Can you work these out from the drawing? Everything is in mm from the part's minimum corner. Give positions to 0.01 mm unless a question says otherwise; leave off trailing zeros. Order: outer loops, then holes, each group sorted by start corner. A loop starts at its lowest first (then second) coordinate and runs counter-clockwise, first axis right, second up. Notation, with made-up numbers: (88.25, 0) -> (133.25, 0) arc R21 ccw to (133.25, 10) -> close; hole circle Ø10 at (-29.5, 83.25). An arc over 180 degrees is marked (long way). Answer as CSV lines item,"result". Start each with the question number.
(1) I want a section at A-A (x = 8.5). Please give me the cut outline in (y, z) (1 decimal).
(2) Will this pin go through, and if not, where does the flat tip stop? pin 1 Ø3.5 at (x, z) = (4.5, 43.5) entering from -Y.
(3) I need wall thicknesses on L1, parallel to Z at x = 9.5, y = 1 (1 decimal); L2, parallel to Z at x = 13.5, y = 0.5 (1 decimal); L3, parallel to X at y = 0.5, z = 50 (1 decimal). Which ranges of each line are inside material? Lowest first, please.
(4) I want a section at C-C (y = 1.6). Give the number of separate pieces and of enclosed holes in the cut face, plus the area to 3 significant figures.
(5) I want a section at B-B (z = 49.5). Please give me the cut outline in (x, y) (1 decimal), plus the area to 3 significant figures.
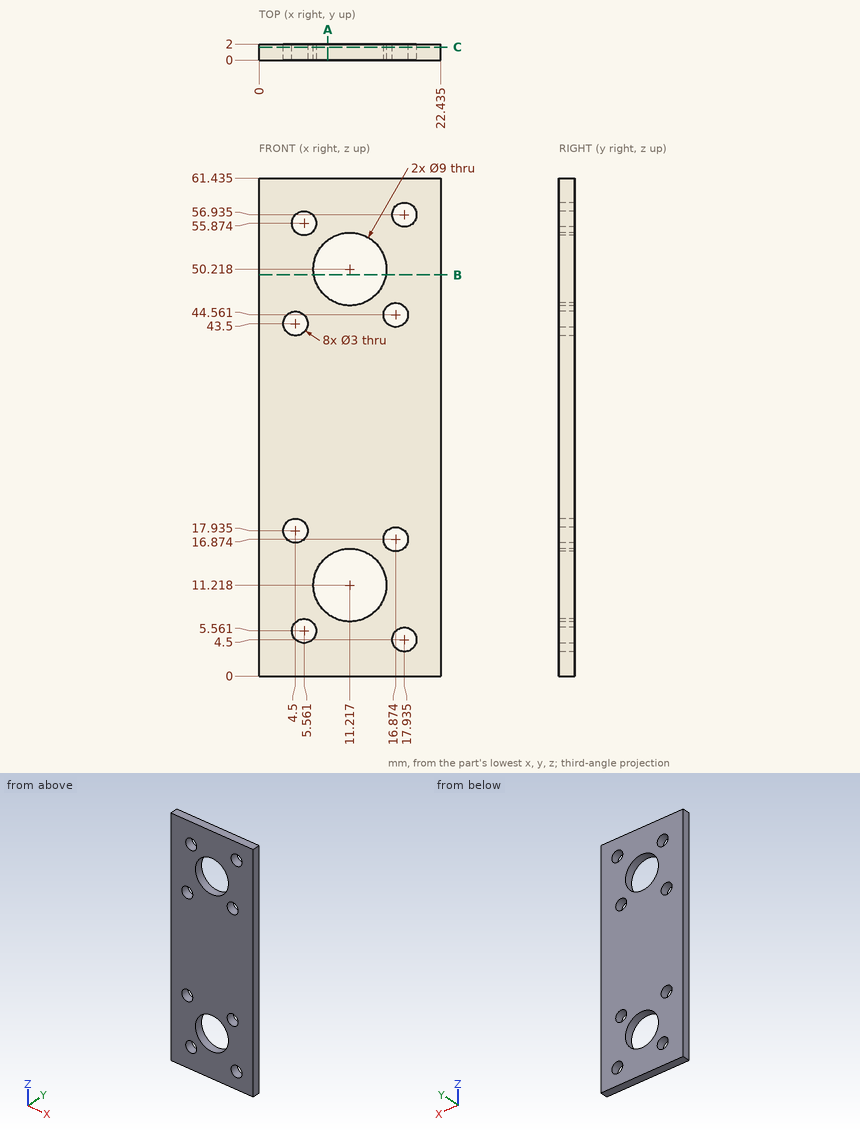
Final values:
1,outline,"(0, 0) -> (2, 0) -> (2, 7.6) -> (0, 7.6) -> close; (0, 14.8) -> (2, 14.8) -> (2, 46.6) -> (0, 46.6) -> close; (0, 53.8) -> (2, 53.8) -> (2, 61.4) -> (0, 61.4) -> close"
2,pin 1,"y = 0"
3,L1,"0 to 7.1, 15.4 to 46.1, 54.4 to 61.4"
3,L2,"0 to 7.3, 15.1 to 46.3, 54.1 to 61.4"
3,L3,"0 to 6.7, 15.7 to 22.4"
4,separate pieces,"1"
4,enclosed holes,"10"
4,area,"1,190 mm²"
5,outline,"(0, 0) -> (6.8, 0) -> (6.8, 2) -> (0, 2) -> close; (15.7, 0) -> (22.4, 0) -> (22.4, 2) -> (15.7, 2) -> close"
5,area,"27.1 mm²"
